Job drawing, mm, ordinate dimensions from the low corner. One solid piece. Give positions to 0.01 mm unless a question says otherwise; leave off trailing zeros. Order: outer loops, then holes, each group sorted by start corner. A loop starts at its lowest first (then second) coordinate and runs counter-clockwise, first axis right, second up.
1. Probe line 1 (Z direction, x = 35, y = 2.5); line 2 (Y direction, x = 37.5, z = 6); line 3 (X direction, y = 50, z = 8.75) (1 decimal). List the from-to ranges inside material, lowest first.
2. Slice it at B-B on y = 49.5. List the corners of the cut face in (x, z).
3. Slice it at D-D on z = 17. List the corners of the cut face in (x, y) (1 decimal), and give its area (3 significant figures).
4. Slice it at C-C on x = 35. List the corners of the cut face in (y, z), and give its area (3 significant figures).
5. Mould opens along X. For the marked faces 1, 2 and 3 say: +X half, -X half, draft (parallel to the pull), parting line (faces both ways), or undercut.
6. Slice it at A-A on z = 10. List the corners of the cut face in (x, y) (1 decimal).
7. Drop flat-ended pins along their axis: pin 1 Ø8 at (y, z) = (31, 16.5) entering from +X (1 decimal); pin 2 Ø1.5 at (y, z) = (3.5, 14) entering from +X; pin 3 Ø8 at (y, z) = (36.5, 17.5) entering from -X; pin 4 Ø11.5 at (x, y) = (104.71, 52) entering from +Z. Give the stop position or say it passes through.
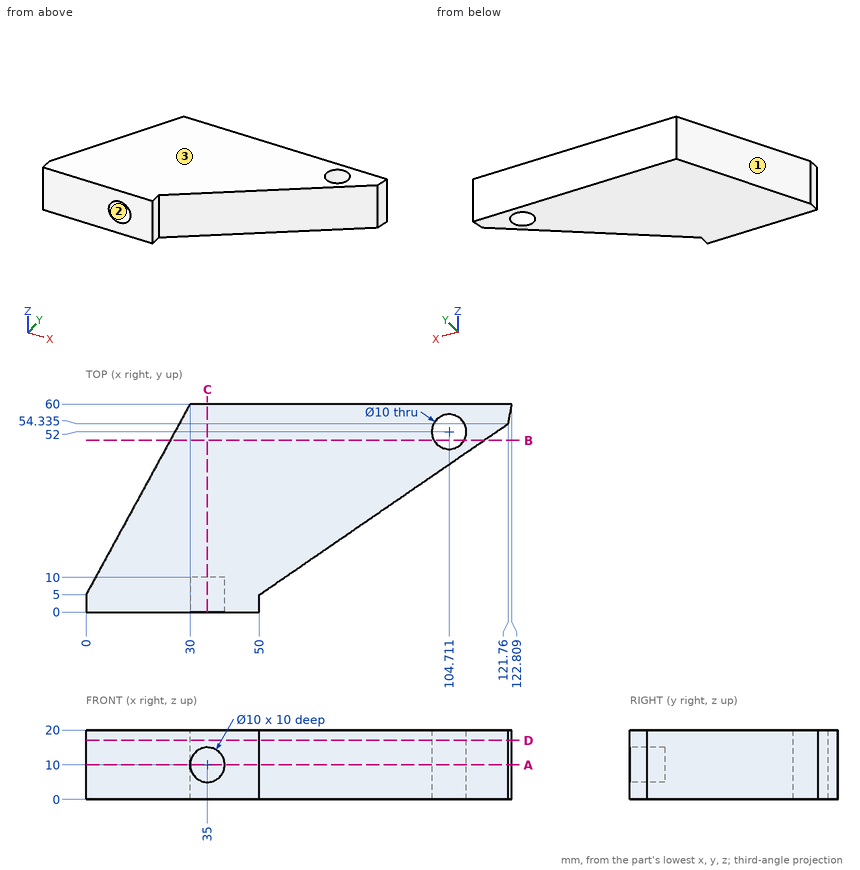
Data:
1. line 1: z = 0 to 5, 15 to 20
1. line 2: y = 10 to 60
1. line 3: x = 24.5 to 100.1, 109.3 to 115.5
2. outline: (24.27, 0) - (100.38, 0) - (100.38, 20) - (24.27, 20) - close; (109.04, 0) - (114.73, 0) - (114.73, 20) - (109.04, 20) - close
3. outline: (0, 0) - (50, 0) - (50, 5) - (121.8, 54.3) - (122.8, 60) - (30, 60) - (0, 5) - close; hole circle Ø10 at (104.7, 52)
3. area: 4,280 mm2
4. outline: (0, 0) - (60, 0) - (60, 20) - (0, 20) - (0, 15) - (10, 15) - (10, 5) - (0, 5) - close
4. area: 1,100 mm2
5. face 1: -X half
5. face 2: undercut
5. face 3: draft
6. outline: (0, 0) - (30, 0) - (30, 10) - (40, 10) - (40, 0) - (50, 0) - (50, 5) - (121.8, 54.3) - (122.8, 60) - (30, 60) - (0, 5) - close; hole circle Ø10 at (104.7, 52)
7. pin 1: stops at x = 93.6
7. pin 2: stops at x = 50
7. pin 3: stops at x = 15
7. pin 4: stops at z = 20
